The listing builds one solid part. Answer for the finished solid, in the listing's coordinates (mm). A direction names the side the tool comes from. Give positions to 0.01 mm unless a question says otherwise; leave off trailing zeros. Write each loop counter-clockwise with the first axis right and the second up, starting at its lowest first coordinate (ties: lowest second). Pieces come first, ordered by that corner, then holes. Notation, with made-up numbers: (10.25, 25.25) - (58.25, 25.25) arc R16 ccw to (58.25, 34.25) - close; hole circle Ø3 at (52, -35). An arc over 180 degrees is marked (long way). Return JSON: item names as keys, results as strings.
from build123d import *

# Parameters (mm, degrees)
PAD_DEPTH    = 10
PAD001_DEPTH = 10


with BuildPart() as part:
    # Sketch → Pad (new body)
    with BuildSketch(Plane.XY):
        with BuildLine():
            Line((7, -1), (-7, -1))
            Line((-7, -1), (-7, 0))
            Line((-7, 0), (-4, 0))
            Line((-4, 13), (-4, 0))
            Line((-3, 13), (-4, 13))
            Line((-3, 0), (-3, 13))
            Line((-3, 0), (6, 0))
            Line((6, 0), (6, 10))
            Line((12, 10), (6, 10))
            ThreePointArc((15, 10), (13.5, 11.5), (12, 10))
            Line((15, 10), (15, 9))
            Line((15, 9), (10, 9))
            Line((10, 9), (10, 8.5))
            ThreePointArc((8.6, 8.5), (9.3, 7.8), (10, 8.5))
            Line((8.6, 9), (8.6, 8.5))
            Line((7, 9), (8.6, 9))
            Line((7, 9), (7, 7.5))
            Line((7, 7.5), (7.5, 7.5))
            ThreePointArc((7.5, 6.5), (8, 7), (7.5, 7.5))
            Line((7, 6.5), (7.5, 6.5))
            Line((7, 6.5), (7, -1))
        make_face()
    extrude(amount=PAD_DEPTH)

    # Sketch → Pad001 (join)
    with BuildSketch(Plane.XY):
        with BuildLine():
            Line((7, -1), (-7, -1))
            Line((-7, -1), (-7, 0))
            Line((-7, 0), (-4, 0))
            Line((-4, 13), (-4, 0))
            Line((-3, 13), (-4, 13))
            Line((-3, 0), (-3, 13))
            Line((-3, 0), (6, 0))
            Line((6, 0), (6, 10))
            Line((12, 10), (6, 10))
            ThreePointArc((15, 10), (13.5, 11.5), (12, 10))
            Line((15, 10), (15, 9))
            Line((15, 9), (10, 9))
            Line((10, 9), (10, 8.5))
            ThreePointArc((8.6, 8.5), (9.3, 7.8), (10, 8.5))
            Line((8.6, 9), (8.6, 8.5))
            Line((7, 9), (8.6, 9))
            Line((7, 9), (7, 7.5))
            Line((7, 7.5), (7.5, 7.5))
            ThreePointArc((7.5, 6.5), (8, 7), (7.5, 7.5))
            Line((7, 6.5), (7.5, 6.5))
            Line((7, 6.5), (7, -1))
        make_face()
    extrude(amount=PAD001_DEPTH)


solid = part.part
Item 1: A cutting plane is placed at C-C on y = 9.5. Determine the outline of the cut face in (x, z), then the cut area to 3 significant figures.
Answer below:
{"outline": "(-4, 0) - (-3, 0) - (-3, 10) - (-4, 10) - close; (6, 0) - (15, 0) - (15, 10) - (6, 10) - close", "area": "100 mm²"}
Item 2: A cutting plane is placed at D-D on x = 13.5. Determine the outline of the cut face in (y, z).
Answer below:
{"outline": "(9, 0) - (11.5, 0) - (11.5, 10) - (9, 10) - close"}
Item 3: A cutting plane is placed at A-A on y = 4.75. Determine the outline of the cut face in (x, z), then the cut area to 3 significant figures.
Answer below:
{"outline": "(-4, 0) - (-3, 0) - (-3, 10) - (-4, 10) - close; (6, 0) - (7, 0) - (7, 10) - (6, 10) - close", "area": "20.0 mm²"}
Item 4: Flat-ended cylindrical pins translate along their axes: P1, Ø1.2, axis at y = 8, z = 5.5, coming from the +X side; P2, Ø1.5, axis at x = -5.5, z = 3, coming from the +Y side; P3, Ø0.6, axis at y = 9, z = 7.5, coming from the -X side; P4, Ø6, axis at x = 1, y = 8.5, coming from the -Z side. Find the tip coordinate at first contact, or state that the pin passes through.
Answer below:
{"P1": "stops at x = 10", "P2": "stops at y = 0", "P3": "stops at x = -4", "P4": "passes through"}
Item 5: For faces 1 (the face through (9.3, 7.8, 4.9)), 2 (the face through (-6, 0, 5)), 3 (the face through (7, 3, 5)), 4 (the face through (9, 10, 5)), 5 (the face through (7, 8, 5)), determine the directions among +Z, -Z, +X, -X, +Y, -Y from which every point of the face is accessible in a straight line to the end or side of a thin tool.
Answer below:
{"face 1": "+Z, -Z, -Y", "face 2": "+Z, -Z, -X, +Y", "face 3": "+Z, -Z, +X, -Y", "face 4": "+Z, -Z, +Y", "face 5": "+Z, -Z"}
Item 6: A cutting plane is placed at B-B on z = 7. Determine the outline of the cut face in (x, y), then the cut area to 3 significant figures.
Answer below:
{"outline": "(-7, -1) - (7, -1) - (7, 6.5) - (7.5, 6.5) arc R0.5 ccw to (7.5, 7.5) - (7, 7.5) - (7, 9) - (8.6, 9) - (8.6, 8.5) arc R0.7 ccw to (10, 8.5) - (10, 9) - (15, 9) - (15, 10) arc R1.5 ccw to (12, 10) - (6, 10) - (6, 0) - (-3, 0) - (-3, 13) - (-4, 13) - (-4, 0) - (-7, 0) - close", "area": "50.9 mm²"}
Item 7: Consider L1, parallel to X at y = 3.5, z = 5.75; L2, parallel to X at y = 8, z = 2.5; L3, parallel to X at y = 8.25, z = 7. Determine where each line is inside the solid, lowest interval first.
Answer below:
{"L1": "x = -4 to -3, 6 to 7", "L2": "x = -4 to -3, 6 to 7, 8.81 to 9.79", "L3": "x = -4 to -3, 6 to 7, 8.65 to 9.95"}
